Source: CAD feature listing. Evaluate the final solid. Frame: model axes, mm. Face numbers are marked on the shaded views. Give positions to 0.01 mm unless a question says otherwise; leave off trailing zeros. Order: outer loops, then holes, each group sorted by start corner. A loop starts at its lowest first (then second) coordinate and runs counter-clockwise, first axis right, second up. Notation, with made-up numbers: M 28.25,65 L 68.25,65 A10 cw 68.25,73 Z; hole C -31,22 d3. An arc over 180 degrees is marked long. Use CSV: the item, a comma, the result in double quotes. Start each with the question number.
1. Section query A-A, the plane y = 0. Return the cut outline in (x, z), plus the area to 3 significant figures.
2. Line query: line 1 along Z through (x, y) = (5, -0.25); line 2 along Y through (x, z) = (16, 0); line 3 along Z through (x, y) = (5.5, -2). Output: solid intervals per line, ascending. Write a range as [from, to].
3. Section query D-D, the plane y = -7.75. Return the cut outline in (x, z), plus the area to 3 significant figures.
4. Mould query, pull axis Y, two halves, no side actions, for the marked faces 1, 2 and 3. Classes: released by +Y, released by -Y, zero draft, split by the parting line, or undercut.
5. Pin query (flat end, axial travel): P1, Ø1, axis at x = 5.5, z = 1.5, coming from the -Y side; P2, Ø2, axis at x = 16.5, y = -3, coming from the +Z side; P3, Ø6, axis at x = 11.5, z = 8.5, coming from the +Y side. Return the tip coordinate at first contact, or that it passes through.
6. Section query C-C, the plane x = 12. Return the cut outline in (y, z).
Autodesk Fusion 360 part; units mm, degrees
sketch "Sketch1" plane through (0, 0, 0) normal (1, 0, 0) x (0, 0, -1)
  circle A0 centre (0, 0) radius 6
  circle A1 centre (0, 0) radius 11
  dimension "d1" = 12
  dimension "d2" = 22
extrude "Extrude1" add sketch "Sketch1" along normal blind 22 makes body 1
copy_body "Body->Comp1" bodies 1 removing the originals makes body 2 in component "12x22x22 bushing"
component "12x22x22 bushing" placed x (1, 0, 0) y (0, 1, 0) z (0, 0, 1) at (0, 0, 0)
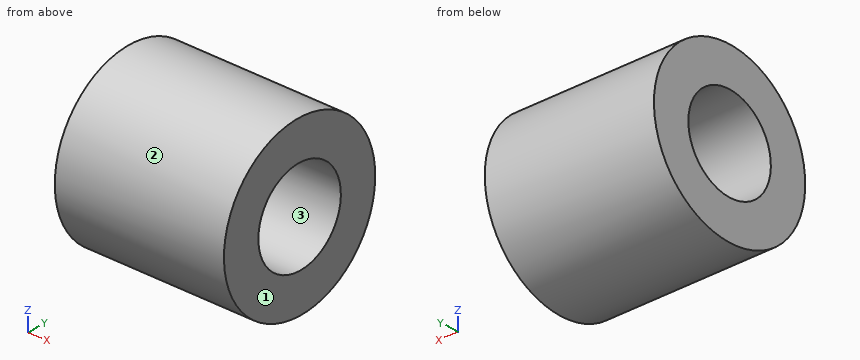
Result set:
1,outline,"M 0,-11 L 22,-11 L 22,-6 L 0,-6 Z; M 0,6 L 22,6 L 22,11 L 0,11 Z"
1,area,"220 mm2"
2,line 1,"[-11, -5.99], [5.99, 11]"
2,line 2,"[-11, -6], [6, 11]"
2,line 3,"[-10.82, -5.66], [5.66, 10.82]"
3,outline,"M 0,-7.81 L 22,-7.81 L 22,7.81 L 0,7.81 Z"
3,area,"343 mm2"
4,face 1,"zero draft"
4,face 2,"split by the parting line"
4,face 3,"undercut"
5,P1,"y = -10.95"
5,P2,"z = 10.82"
5,P3,"y = 9.53"
6,outline,"C 0,0 d22; hole C 0,0 d12"
